Autodesk Inventor part; units mm, degrees
ref_plane "YZ Plane" through (0, 0, 0) normal (1, 0, 0) x (0, 1, 0)
ref_plane "XZ Plane" through (0, 0, 0) normal (0, 1, 0) x (-1, 0, 0)
ref_plane "XY Plane" through (0, 0, 0) normal (0, 0, 1) x (1, 0, 0)
ref_plane "Work Plane1" through (3.4455, 2.6204, 52.7) normal (0, 0, 1) x (1, 0, 0)
sketch "Sketch1" plane through (3.4455, 2.6204, 52.7) normal (0, 0, 1) x (1, 0, 0)
  circle A0 centre (0, 0) radius 1.5
  line L0 (-5.25, 4.25) -> (5.25, 4.25)
  line L1 (5.25, 4.25) -> (5.25, -5.25)
  line L2 (5.25, -5.25) -> (-5.25, -5.25)
  line L3 (-5.25, -5.25) -> (-5.25, 4.25)
  point P0 (-3.4455, -2.6204)
  dimension "d2" = 10.5
  dimension "d4" = 4.25
  dimension "d6" = 5.25
  dimension "d7" = 9.5
extrude "Extrusion1" add sketch "Sketch1" along normal blind 1.15
sketch "Sketch2" plane through (3.4455, 2.6204, 52.7) normal (0, 0, -1) x (-1, 0, 0)
  line L0 (-5.25, 4.25) -> (-5.25, -5.25)
  line L1 (-5.25, -5.25) -> (5.25, -5.25)
  line L2 (5.25, -5.25) -> (5.25, 4.25)
  line L3 (-5.25, -5.25) -> (-5.25, -4.1)
  line L4 (-5.25, -4.1) -> (5.25, -4.1)
  point P0 (3.4455, -2.6204)
  dimension "d10" = 1.15
extrude "Extrusion2" add sketch "Sketch2" along normal blind 1.5
sketch "Sketch3" plane through (-1.8045, -2.6296, 53.85) normal (0, -1, 0) x (1, 0, 0)
  line L0 (0, 0) -> (10.5, 0)
  line L1 (10.5, -2.65) -> (0, -2.65)
  line L2 (5.25, -54.5) -> (12.75, -54.5)
  line L3 (5.25, 0) -> (5.25, -54.5) construction
  line L4 (12.75, -54.5) -> (12.75, -47.5)
  line L5 (10.5, -10) -> (10.5, -44.5)
  line L6 (12.75, -2.65) -> (12.75, -8)
  line L7 (5.25, -2.65) -> (12.75, -2.65)
  line L8 (12.75, -8) -> (10.5, -10)
  line L9 (10.5, -44.5) -> (12.75, -47.5)
  line L10 (5.25, -54.5) -> (-2.25, -54.5)
  line L11 (-2.25, -54.5) -> (-2.25, -47.5)
  line L12 (0, -10) -> (0, -44.5)
  line L13 (-2.25, -2.65) -> (-2.25, -8)
  line L14 (5.25, -2.65) -> (-2.25, -2.65)
  line L15 (-2.25, -8) -> (0, -10)
  line L16 (0, -44.5) -> (-2.25, -47.5)
  circle A0 centre (5.25, -5.75) radius 1.125
  circle A1 centre (0.75, -5.75) radius 1.125
  circle A2 centre (9.75, -5.75) radius 1.125
  circle A3 centre (0.75, -49.75) radius 1.125
  circle A4 centre (9.75, -49.75) radius 1.125
  circle A5 centre (5.25, -49.75) radius 1.125
  dimension "d13" = 54.5
  dimension "d15" = 7.5
  dimension "d16" = 7
  dimension "d17" = 10
  dimension "d18" = 34.5
  dimension "d19" = 5.25
  dimension "d20" = 8
  dimension "d21" = 7.5
  dimension "d24" = 2.25
  dimension "d25" = 5.75
  dimension "d26" = 2.25
  dimension "d27" = 4.5
  dimension "d28" = 2.25
  dimension "d29" = 4.5
  dimension "d30" = 4.75
  dimension "d32" = 5.75
  dimension "d33" = 4.5
  dimension "d34" = 2.25
  dimension "d35" = 2.25
  dimension "d36" = 2.25
extrude "Extrusion3" add sketch "Sketch3" against normal blind 1.15
sketch "Sketch4" plane through (10.9455, -2.6296, -0.65) normal (0, 0, -1) x (-1, 0, 0)
  line L0 (2.25, 1.15) -> (12.75, 1.15)
  line L1 (12.75, 1.15) -> (12.75, 9.5)
  line L2 (12.75, 9.5) -> (2.25, 9.5)
  line L3 (2.25, 9.5) -> (2.25, 1.15)
  circle A0 centre (7.5, 5.25) radius 1.5
  line L4 (0, 1.15) -> (0, 5.25)
  line L5 (15, 1.15) -> (15, 5.25)
  line L6 (0, 1.15) -> (15, 1.15)
  circle A1 centre (7.5, 5.25) radius 1.5
  arc A2 (1.2199, 1.15) -> (13.7801, 1.15) centre (7.5, 5.25) ccw
  arc A3 (15, 5.25) -> (0, 5.25) centre (7.5, 5.25) ccw
  point P0 (10.9455, 2.6296)
extrude "Extrusion4" add sketch "Sketch4" against normal blind 1.15 contours L3 L2 L1 L0 | L6 L4 A3 L5 L1 L2 L3
Part model, mm, in its own coordinate system. A direction names the side the tool comes from. Round coordinates to 2 decimals unless told otherwise and drop trailing zeros. Loops run counter-clockwise (first coordinate to the right, second up) from the corner with the lowest first, then second, coordinate; pieces in that order, holes last. Notation, with made-up numbers: (40, -16) - (65, -16) arc R8 cw to (65, -1) - close; hole circle Ø11 at (28, 5.25). An arc over 180 degrees is marked (long way). Answer as a JSON object with one key per item and string values.
Item 1: Band-saw the part on C-C on y = 4.75. List the corners of the cut face in (x, z).
Output:
{"outline": "(-3.75, -0.65) - (10.64, -0.65) - (10.64, 0.5) - (-3.75, 0.5) - close; (-1.8, 52.7) - (8.7, 52.7) - (8.7, 53.85) - (-1.8, 53.85) - close"}
Item 2: Band-saw the part on A-A on z = 48.1. List the corners of the cut face in (x, y), plus the area to 3 significant figures.
Output:
{"outline": "(-4.05, -2.63) - (-2.18, -2.63) - (-2.18, -1.48) - (-4.05, -1.48) - close; (0.07, -2.63) - (2.32, -2.63) - (2.32, -1.48) - (0.07, -1.48) - close; (4.57, -2.63) - (6.82, -2.63) - (6.82, -1.48) - (4.57, -1.48) - close; (9.07, -2.63) - (10.95, -2.63) - (10.95, -1.48) - (9.07, -1.48) - close", "area": "9.49 mm2"}
Item 3: Pin check, flat tips, straight feed: pin 1 (1.3 mm diameter, centred on x = 4, z = 53.5, fed in from +Y); pin 2 (0.6 mm diameter, centred on y = -2, z = 30.5, fed in from -X); pin 3 (2.5 mm diameter, centred on x = 3.45, z = 48.1, fed in from +Y). Stop position of each tip, or through.
Output:
{"pin 1": "y = 6.87", "pin 2": "x = -1.8", "pin 3": "y = -1.48"}
Item 4: Band-saw the part on B-B on x = -1. List the corners of the cut face in (y, z), plus the area to 3 significant figures.
Output:
{"outline": "(-2.63, -0.65) - (8.66, -0.65) - (8.66, 0.5) - (-1.48, 0.5) - (-1.48, 2.98) - (-2.63, 2.98) - close; (-2.63, 5.22) - (-1.48, 5.22) - (-1.48, 46.98) - (-2.63, 46.98) - close; (-2.63, 49.22) - (-1.48, 49.22) - (-1.48, 52.7) - (6.87, 52.7) - (6.87, 53.85) - (-2.63, 53.85) - close", "area": "78.8 mm2"}
Item 5: Band-saw the part on D-D on x = 3. List the corners of the cut face in (y, z).
Output:
{"outline": "(-2.63, -0.65) - (1.19, -0.65) - (1.19, 0.5) - (-1.48, 0.5) - (-1.48, 3.07) - (-2.63, 3.07) - close; (-2.63, 5.13) - (-1.48, 5.13) - (-1.48, 47.07) - (-2.63, 47.07) - close; (-2.63, 49.13) - (-1.48, 49.13) - (-1.48, 52.7) - (1.19, 52.7) - (1.19, 53.85) - (-2.63, 53.85) - close; (4.05, -0.65) - (10.11, -0.65) - (10.11, 0.5) - (4.05, 0.5) - close; (4.05, 52.7) - (6.87, 52.7) - (6.87, 53.85) - (4.05, 53.85) - close"}
Item 6: Tool access for faces 1 (the face through (9.836, -2.063, 44.864)), 2 (the face through (-1.804, -2, 27)), 3 (the face through (3.6, 4.4, 0.5)), 4 (the face through (8.696, 2, 53)): list every direction of +Z, -Z, +X, -X, +Y, -Y with a clear straight run to the whole face (end or side of a thin tool).
Output:
{"face 1": "+X, +Y, -Y", "face 2": "-X, +Y, -Y", "face 3": "+X, -X, +Y", "face 4": "+Z, +X, +Y, -Y"}
Item 7: Pull direction X, two halves, no side cores. Call faces 5 (the face through (3.96, -2.06, 3.1)), 6 (the face through (3, 6.87, 53)), 7 (the face through (3.28, 10.12, -0.08)): pulls with the +X half, pulls with the -X half, needs draft (parallel to the pull), parting line crosses it, or undercut.
Output:
{"face 5": "undercut", "face 6": "needs draft", "face 7": "parting line crosses it"}
Item 8: Wall check: L1, parallel to Z at x = 8, y = -1.75; L2, parallel to Z at x = 6.25, y = 3; L3, parallel to Y at x = 0.25, z = 17.5. Give the ranges that are in metal, low to high.
Output:
{"L1": "-0.65 to 2.98, 5.22 to 46.98, 49.22 to 53.85", "L2": "-0.65 to 0.5, 52.7 to 53.85", "L3": "-2.63 to -1.48"}
